```python
from build123d import *

# Parameters (mm, degrees)
SCHIZZO2_W                   = 5.93
SCHIZZO2_H                   = 25
ESTRUSIONE_ESTRUSIONE1_DEPTH = 83.26
SCHIZZO3_W                   = 2
SCHIZZO3_H                   = 25
ESTRUSIONE_ESTRUSIONE2_DEPTH = 7
SCHIZZO4_W                   = 1
SCHIZZO4_H                   = 25
ESTRUSIONE_ESTRUSIONE3_DEPTH = 5
SCHIZZO5_W                   = 1
SCHIZZO5_H                   = 25
ESTRUSIONE_ESTRUSIONE4_DEPTH = 6
SCHIZZO7_W                   = 5.93
SCHIZZO7_H                   = 25
ESTRUSIONE_ESTRUSIONE5_DEPTH = 3.83
SCHIZZO9_W                   = 3.83
SCHIZZO9_H                   = 25
ESTRUSIONE_ESTRUSIONE7_DEPTH = 12.34


with BuildPart() as part:
    # Schizzo2 → Estrusione-Estrusione1 (new body)
    with BuildSketch(Plane.XY):
        with Locations((0, 12.5)):
            Rectangle(SCHIZZO2_W, SCHIZZO2_H)
    extrude(amount=-ESTRUSIONE_ESTRUSIONE1_DEPTH)

    # Schizzo3 → Estrusione-Estrusione2 (add)
    with BuildSketch(Plane(origin=(2.965, 0, 0), x_dir=(0, 0, -1), z_dir=(1, 0, 0))):
        with Locations((82.26, 12.5)):
            Rectangle(SCHIZZO3_W, SCHIZZO3_H)
    extrude(amount=ESTRUSIONE_ESTRUSIONE2_DEPTH)

    # Schizzo4 → Estrusione-Estrusione3 (add)
    with BuildSketch(Plane.XY.offset(-81.26)):
        with Locations((9.465, 12.5)):
            Rectangle(SCHIZZO4_W, SCHIZZO4_H)
    extrude(amount=ESTRUSIONE_ESTRUSIONE3_DEPTH)

    # Schizzo5 → Estrusione-Estrusione4 (add)
    with BuildSketch(Plane.ZY.offset(-8.965)):
        with Locations((-76.76, 12.5)):
            Rectangle(SCHIZZO5_W, SCHIZZO5_H)
    extrude(amount=ESTRUSIONE_ESTRUSIONE4_DEPTH)

    # Schizzo7 → Estrusione-Estrusione5 (add)
    with BuildSketch(Plane.XY):
        with Locations((0, 12.5)):
            Rectangle(SCHIZZO7_W, SCHIZZO7_H)
    extrude(amount=ESTRUSIONE_ESTRUSIONE5_DEPTH)

    # Schizzo9 → Estrusione-Estrusione7 (add)
    with BuildSketch(Plane(origin=(2.965, 0, 0), x_dir=(0, 0, -1), z_dir=(1, 0, 0))):
        with Locations((-1.915, 12.5)):
            Rectangle(SCHIZZO9_W, SCHIZZO9_H)
    extrude(amount=ESTRUSIONE_ESTRUSIONE7_DEPTH)


solid = part.part
```
The model under review builds one solid part; all positions refer to its coordinate system, in mm. A direction names the side the tool comes from. Give positions to 0.01 mm unless a question says otherwise; leave off trailing zeros. Write each loop counter-clockwise with the first axis right and the second up, starting at its lowest first coordinate (ties: lowest second). Pieces come first, ordered by that corner, then holes.
(1) For P1, Ø10, axis at y = 4, z = -20.5, coming from the +X side (3 decimals); P2, Ø2, axis at y = 10, z = -78.5, coming from the +X side (3 decimals), all flat-tipped, find the tip position at first contact; note any pin that passes through.
(2) Consider section B-B, the plane y = 23.25. Give the boundary of the cut face in (x, z) (3 decimals), and give its area (3 significant figures).
(3) Consider section C-C, the plane x = 12.5. Give the boundary of the cut face in (y, z), and give its area (4 significant figures).
(4) Consider section D-D, the plane z = -47. Give the boundary of the cut face in (x, y) (3 decimals).
(5) Consider section A-A, the plane x = 6.5. Give the boundary of the cut face in (y, z), and give its area (3 significant figures).
(6) Tool access review of faces 4 (the flat face through (-2.965, 12, -40)), 5 (the flat face through (8.965, 12, -79)), 6 (the flat face through (9.965, 12, -80)), 7 (the flat face through (7, 12, -76.26)): name each direction out of +Z, -Z, +X, -X, +Y, -Y from which nothing blocks a thin tool from reaching the whole face with its end or side.
(7) The part is to be moulded in two halves that separate along Z. For faces 1 (the flat face through (15.305, 13, 2)), 2 (the flat face through (3, 12, -83.26)), 3 (the flat face through (6, 12, -81.26)), say which applies: released by +Z, released by -Z, zero draft, split by the parting line, or undercut.
(8) To check wall thickness, follow L1, parallel to Z at x = 7, y = 20.5; L2, parallel to X at y = 10.25, z = -38 (3 decimals); L3, parallel to Z at x = 12.5, y = 1.5. State the ranges of each line that lie inside material, in increasing order.
Returned:
1. P1: stops at x = 2.965
1. P2: stops at x = 9.965
2. outline: (-2.965, -83.26) - (9.965, -83.26) - (9.965, -76.26) - (2.965, -76.26) - (2.965, 0) - (15.305, 0) - (15.305, 3.83) - (-2.965, 3.83) - close; hole (2.965, -81.26) - (8.965, -81.26) - (8.965, -77.26) - (2.965, -77.26) - close
2. area: 589 mm2
3. outline: (0, 0) - (25, 0) - (25, 3.83) - (0, 3.83) - close
3. area: 95.75 mm2
4. outline: (-2.965, 0) - (2.965, 0) - (2.965, 25) - (-2.965, 25) - close
5. outline: (0, -83.26) - (25, -83.26) - (25, -81.26) - (0, -81.26) - close; (0, -77.26) - (25, -77.26) - (25, -76.26) - (0, -76.26) - close; (0, 0) - (25, 0) - (25, 3.83) - (0, 3.83) - close
5. area: 171 mm2
6. face 4: +Z, -Z, -X, +Y, -Y
6. face 5: +Y, -Y
6. face 6: -Z, +X, +Y, -Y
6. face 7: +X, +Y, -Y
7. face 1: zero draft
7. face 2: released by -Z
7. face 3: undercut
8. L1: z = -83.26 to -81.26, -77.26 to -76.26, 0 to 3.83
8. L2: x = -2.965 to 2.965
8. L3: z = 0 to 3.83
